Part model, mm, in its own coordinate system. A direction names the side the tool comes from. Round coordinates to 2 decimals unless told otherwise and drop trailing zeros. Write each loop counter-clockwise with the first axis right and the second up, starting at its lowest first coordinate (ties: lowest second). Pieces come first, ordered by that corner, then holes. Notation, with made-up numbers: (-19.75, -15) -> (0.25, -15) arc R13 ccw to (0.25, -11) -> close; hole circle Ø10 at (33, 30). An arc over 180 degrees is marked (long way). Use CSV: the item, a comma, the result in double quotes. Start each with the question number.
(1) Saw through at B-B (y = 0). Give the cut face in (x, z).
(2) Two-plate mould, pull along Y, no slides. Class faces 1 (the cylindrical face through (6.3, -4.3, 2.5)), 2 (the cylindrical face through (11.923, 3.755, 2.465)), 3 (the flat face through (-0.1, -2.2, 8)): released by +Y, released by -Y, zero draft, split by the parting line, or undercut.
(3) Saw through at C-C (z = 1.5). Give the cut face in (x, y).
(4) Drop flat-ended pins along their axis: pin 1 (4 mm diameter, centred on x = 8.5, y = -4, fed in from +Z); pin 2 (2 mm diameter, centred on x = -7.5, z = 5.5, fed in from -Y); pin 3 (1.5 mm diameter, centred on x = -3, z = 4, fed in from -Y); pin 4 (2.5 mm diameter, centred on x = -5.66, y = -5.66, fed in from -Z). Give the stop position or say it passes through.
(5) Saw through at D-D (x = 10). Give the cut face in (y, z), plus the area to 3 significant figures.
(6) Saw through at A-A (x = 0). Give the cut face in (y, z).
(7) Which spindle directions (+Z, -Z, +X, -X, +Y, -Y) get a long thin tool onto all of the face, cutting with end or side? Do faces 4 (the flat face through (0, -3, 0)), 5 (the cylindrical face through (-1.08, -4.88, 6.48)), 6 (the flat face through (0, 1.323, 2)). Say none if no direction does.
(8) Probe line 1 (X direction, y = 5, z = 2.25); line 2 (Y direction, x = -6.5, z = 1). List the from-to ranges inside material, lowest first. Write a range as [from, to].
```python
from build123d import *

# Parameters (mm, degrees)
F0_R     = 12.5
F1_DEPTH = 5
F2_R     = 5
F3_DEPTH = 3
F4_R     = 2
F5_DEPTH = 3
F7_DEPTH = 25
F8_R     = 1.5
F9_DEPTH = 25


with BuildPart() as f1:
    # F0 (on Top) → F1 (new body)
    with BuildSketch(Plane.XY):
        Circle(F0_R)
    extrude(amount=F1_DEPTH)

    # F2 (on face) → F3 (join)
    with BuildSketch(Plane.XY.offset(5)):
        Circle(F2_R)
    extrude(amount=F3_DEPTH)

    # F4 (on face) → F5 (cut)
    with BuildSketch(Plane.XY.offset(8)):
        Circle(F4_R)
    extrude(amount=-F5_DEPTH, mode=Mode.SUBTRACT)

    # F6 (on face) → F7 (cut)
    with BuildSketch(Plane(origin=(0, 0, 0), x_dir=(1, 0, 0), z_dir=(0, 0, -1))):
        with BuildLine():
            Line((-1.5, -1.3228756555), (1.5, -1.3228756555))
            ThreePointArc((1.5, -1.3228756555), (0, 2), (-1.5, -1.3228756555))
        make_face()
    extrude(amount=-F7_DEPTH, mode=Mode.SUBTRACT)

    # F8 (on face) → F9 (cut)
    with BuildSketch(Plane(origin=(0, 0, 0), x_dir=(1, 0, 0), z_dir=(0, 0, -1))):
        with Locations((-5.6568542495, 5.6568542495)):
            Circle(F8_R)
        with Locations((-5.6568542495, -5.6568542495)):
            Circle(F8_R)
        with Locations((5.6568542495, -5.6568542495)):
            Circle(F8_R)
        with Locations((5.6568542495, 5.6568542495)):
            Circle(F8_R)
    extrude(amount=-F9_DEPTH, mode=Mode.SUBTRACT)


solid = f1.part
```
Answers:
1,outline,"(-12.5, 0) -> (-2, 0) -> (-2, 8) -> (-5, 8) -> (-5, 5) -> (-12.5, 5) -> close; (2, 0) -> (12.5, 0) -> (12.5, 5) -> (5, 5) -> (5, 8) -> (2, 8) -> close"
2,face 1,"undercut"
2,face 2,"split by the parting line"
2,face 3,"zero draft"
3,outline,"circle Ø25 at (0, 0); hole circle Ø3 at (-5.66, -5.66); hole circle Ø3 at (-5.66, 5.66); hole (-1.5, 1.32) arc R2 ccw (long way) to (1.5, 1.32) -> close; hole circle Ø3 at (5.66, -5.66); hole circle Ø3 at (5.66, 5.66)"
4,pin 1,"stops at z = 5"
4,pin 2,"stops at y = -10.59"
4,pin 3,"stops at y = -12.3"
4,pin 4,"passes through"
5,outline,"(-7.5, 0) -> (7.5, 0) -> (7.5, 5) -> (-7.5, 5) -> close"
5,area,"75.0 mm²"
6,outline,"(-12.5, 0) -> (-2, 0) -> (-2, 8) -> (-5, 8) -> (-5, 5) -> (-12.5, 5) -> close; (1.32, 0) -> (12.5, 0) -> (12.5, 5) -> (5, 5) -> (5, 8) -> (2, 8) -> (2, 5) -> (1.32, 5) -> close"
7,face 4,"-Z, +X, -X, +Y, -Y"
7,face 5,"+Z"
7,face 6,"+Z, -Z"
8,line 1,"x = [-11.46, -7.01], [-4.31, 4.31], [7.01, 11.46]"
8,line 2,"y = [-10.68, -6.9], [-4.42, 4.42], [6.9, 10.68]"
